Could you check a few things on this drawing? It's one solid part, dimensions in mm from its lowest x, y, z. Give positions to 0.01 mm unless a question says otherwise; leave off trailing zeros. Order: outer loops, then holes, each group sorted by start corner. A loop starts at its lowest first (then second) coordinate and runs counter-clockwise, first axis right, second up. Notation, with made-up numbers: M -40,-17 L -12,-17 A8 ccw -12,-7 Z; hole C 3,35.5 d9. An arc over 180 degrees is marked long. Use one line per item in the form item = value.
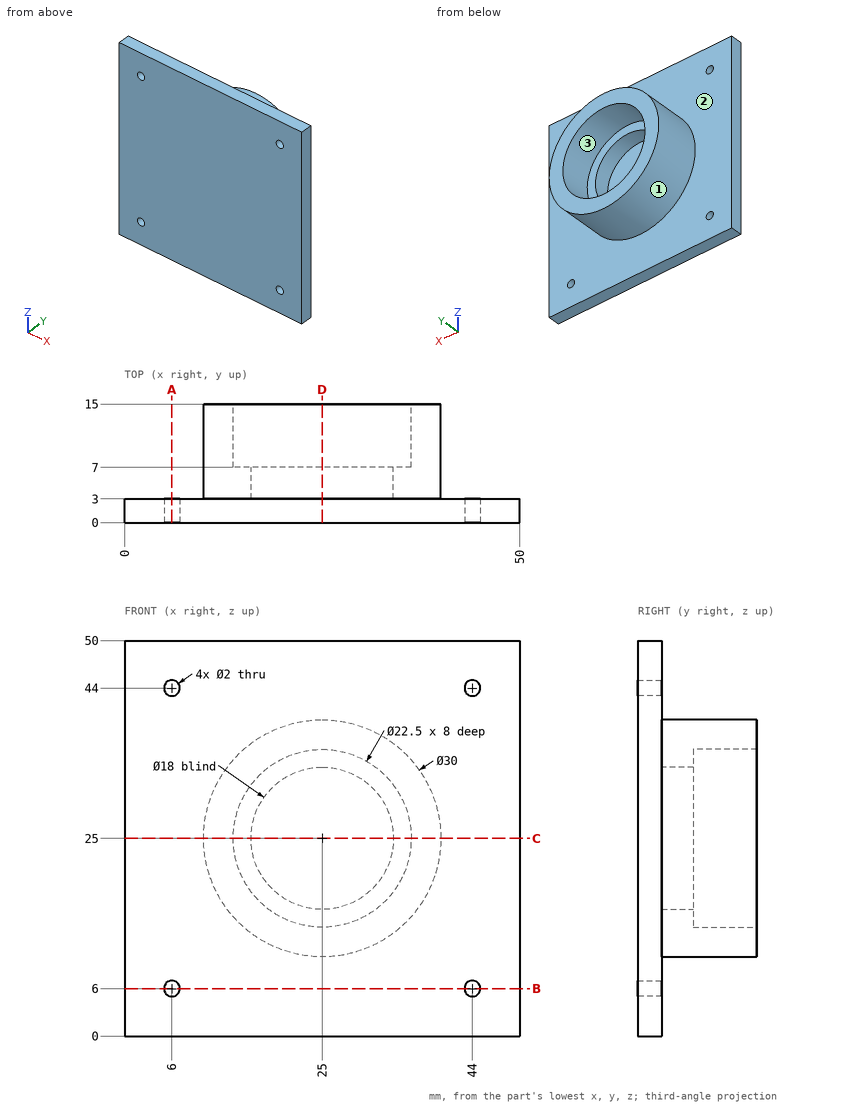
Q1. Thinking about a two-plate mould opening in X: for the marked faces 1, 2 and 3, which applies, +X half, -X half, draft (parallel to the pull), parting line (faces both ways), or undercut?
Found:
face_1 = parting line
face_2 = draft
face_3 = undercut
Q2. I need wall thicknesses on L1, parallel to X at y = 2.3, z = 44; L2, parallel to X at y = 10, z = 25; L3, parallel to X at y = 6.05, z = 25. Which ranges of each line are inside material? Lowest first, please.
Found:
L1 = 0 to 5, 7 to 43, 45 to 50
L2 = 10 to 13.75, 36.25 to 40
L3 = 10 to 16, 34 to 40
Q3. I want a section at B-B on z = 6. Write out the boundary of the cut face in (x, y).
Found:
outline = M 0,0 L 5,0 L 5,3 L 0,3 Z; M 7,0 L 43,0 L 43,3 L 7,3 Z; M 45,0 L 50,0 L 50,3 L 45,3 Z
Q4. I want a section at A-A on x = 6. Write out the boundary of the cut face in (y, z).
Found:
outline = M 0,0 L 3,0 L 3,5 L 0,5 Z; M 0,7 L 3,7 L 3,43 L 0,43 Z; M 0,45 L 3,45 L 3,50 L 0,50 Z
Q5. I'm going to push flat-ended pins straight in: pin 1 Ø6 at (x, y) = (43.5, 9) entering from -Z; pin 2 Ø1 at (y, z) = (4, 38) entering from +X; pin 3 Ø5 at (y, z) = (11.5, 33.5) entering from -X; pin 4 Ø5 at (y, z) = (12.5, 20) entering from +X. Where does each tip first touch, or does it pass through?
Found:
pin_1 = through
pin_2 = 33.29
pin_3 = 11.25
pin_4 = 39.79
Q6. I want a section at C-C on z = 25. Write out the boundary of the cut face in (x, y).
Found:
outline = M 0,0 L 50,0 L 50,3 L 40,3 L 40,15 L 36.25,15 L 36.25,7 L 34,7 L 34,3 L 16,3 L 16,7 L 13.75,7 L 13.75,15 L 10,15 L 10,3 L 0,3 Z
Q7. I want a section at D-D on x = 25. Write out the boundary of the cut face in (y, z), then the cut area to 3 significant figures.
Found:
outline = M 0,0 L 3,0 L 3,10 L 15,10 L 15,13.75 L 7,13.75 L 7,16 L 3,16 L 3,34 L 7,34 L 7,36.25 L 15,36.25 L 15,40 L 3,40 L 3,50 L 0,50 Z
area = 258 mm²
